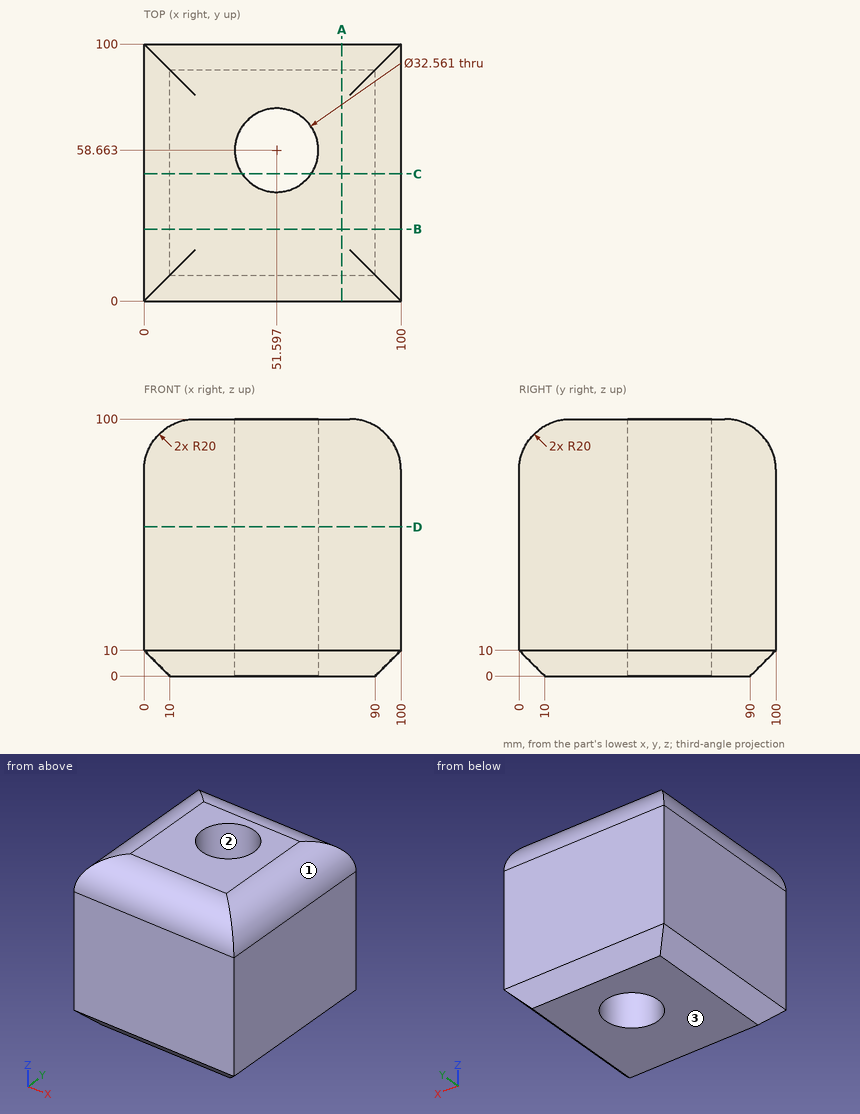
Source: three-view drawing plus pictorial views. Frame: mm from the lowest corner of the part. Coordinates: 2 decimals unless noted, no trailing zeros. Order: outer loops, then holes, each group sorted by start corner. A loop starts at its lowest first (then second) coordinate and runs counter-clockwise, first axis right, second up. Notation, with made-up numbers: M 25.25,70 L 65.25,70 A16 ccw 65.25,76 Z; hole C 58.5,57 d10. An arc over 180 degrees is marked long. Answer in a Markdown table with one row per item.
(1) Section query A-A, the plane x = 77. Output: boundary loops of the cut face in (y, z).
Numbers:
| item | result |
|---|---|
| outline | M 0,10 L 10,0 L 90,0 L 100,10 L 100,80 A20 ccw 80,100 L 20,100 A20 ccw 0,80 Z |
(2) Section query C-C, the plane y = 49.5. Output: boundary loops of the cut face in (x, z) (1 decimal).
Numbers:
| item | result |
|---|---|
| outline | M 0,10 L 10,0 L 38.1,0 L 38.1,100 L 20,100 A20 ccw 0,80 Z; M 65.1,0 L 90,0 L 100,10 L 100,80 A20 ccw 80,100 L 65.1,100 Z |
(3) Section query D-D, the plane z = 58. Output: boundary loops of the cut face in (x, y).
Numbers:
| item | result |
|---|---|
| outline | M 0,0 L 100,0 L 100,100 L 0,100 Z; hole C 51.6,58.66 d32.56 |
(4) Contact query for flat-ended pins moving along their axis: pin 1 Ø6 at (x, y) = (22, 85.5) entering from +Z; pin 2 Ø1 at (x, z) = (82, 88.5) entering from +Y. Output: stop coordinate, or through.
Numbers:
| item | result |
|---|---|
| pin 1 | stops at z = 99.84 |
| pin 2 | stops at y = 98.33 |
(5) Material intervals for line 1 (X direction, y = 64, z = 33.5); line 2 (Y direction, x = 49.5, z = 22); line 3 (Y direction, x = 54.5, z = 83), sorted ascending. Write a range as [from, to].
Numbers:
| item | result |
|---|---|
| line 1 | x = [0, 36.22], [66.98, 100] |
| line 2 | y = [0, 42.52], [74.81, 100] |
| line 3 | y = [0.23, 42.64], [74.68, 99.77] |
(6) Draft query along X for the marked faces 1, 2 and 3. Return one class per face: pulls with the +X half, pulls with the -X half, needs draft (parallel to the pull), parting line crosses it, or undercut.
Numbers:
| item | result |
|---|---|
| face 1 | pulls with the +X half |
| face 2 | undercut |
| face 3 | needs draft |
